from build123d import *

# Parameters (mm, degrees)
BOSS_EXTRUDE1_DEPTH = 7.6
SKETCH2_W           = 36.6
SKETCH2_H           = 8
BOSS_EXTRUDE2_DEPTH = 7.4
SKETCH3_R           = 2
CUT_EXTRUDE1_DEPTH  = 81.259594442
SKETCH4_R           = 2
CUT_EXTRUDE2_DEPTH  = 80.210873622


with BuildPart() as part:
    # Sketch1 → Boss-Extrude1 (new body)
    with BuildSketch(Plane.XY):
        with BuildLine():
            Line((57.05, 42), (41.05, 42))
            Line((41.05, 42), (37, 46.05))
            Line((37, 46.05), (34, 46.05))
            Line((34, 46.05), (32.25, 44.718087488))
            Line((32.25, 44.718087488), (32.25, 25.468087488))
            ThreePointArc((32.25, 25.468087488), (24.422154993, 14.809809015), (11.91, 19.09))
            Line((11.91, 19.09), (10, 21))
            Line((10, 21), (5, 21))
            Line((5, 21), (0, 16))
            Line((0, 16), (0, 0))
            Line((0, 0), (27.4, 0))
            Line((27.4, 0), (27.4, -8))
            Line((27.4, -8), (64, -8))
            Line((64, -8), (64, 35.05))
            Line((64, 35.05), (57.05, 42))
        make_face()
    extrude(amount=BOSS_EXTRUDE1_DEPTH)

    # Sketch2 → Boss-Extrude2 (add)
    with BuildSketch(Plane.XY.offset(7.6)):
        with Locations((45.7, -4)):
            Rectangle(SKETCH2_W, SKETCH2_H)
    extrude(amount=BOSS_EXTRUDE2_DEPTH)

    # Sketch3 → Cut-Extrude1 (cut, through all)
    with BuildSketch(Plane(origin=(0, 0, 0), x_dir=(1, 0, 0), z_dir=(0, 1, 0))):
        with Locations(Location((54, -11, 0), (0, 0, 270))):
            Circle(SKETCH3_R)
        with Locations(Location((34, -11, 0), (0, 0, 270))):
            Circle(SKETCH3_R)
    extrude(amount=-CUT_EXTRUDE1_DEPTH, mode=Mode.SUBTRACT)

    # Sketch4 → Cut-Extrude2 (cut, through all)
    with BuildSketch(Plane.XY.offset(7.6)):
        with Locations((5.08, 9.968087488)):
            Circle(SKETCH4_R)
        with Locations((36.08, 40.968087488)):
            Circle(SKETCH4_R)
    extrude(amount=-CUT_EXTRUDE2_DEPTH, mode=Mode.SUBTRACT)


solid = part.part
Read the model definition and answer for the solid it produces. Units are mm, in the model's axes. A direction names the side the tool comes from. Coordinates: 2 decimals unless noted, no trailing zeros. Loops run counter-clockwise (first coordinate to the right, second up) from the corner with the lowest first, then second, coordinate; pieces in that order, holes last. Notation, with made-up numbers: (-36, 23) -> (-7, 23) arc R21 cw to (-7, 30) -> close; hole circle Ø2 at (32, 58.25). An arc over 180 degrees is marked (long way). Answer in a Markdown table with one row per item.
Item 1: A cutting plane is placed at C-C on z = 6. Determine the outline of the cut face in (x, y), plus the area to 3 significant figures.
Returned:
| item | result |
|---|---|
| outline | (0, 0) -> (27.4, 0) -> (27.4, -8) -> (64, -8) -> (64, 35.05) -> (57.05, 42) -> (41.05, 42) -> (37, 46.05) -> (34, 46.05) -> (32.25, 44.72) -> (32.25, 25.47) arc R11.17 cw to (11.91, 19.09) -> (10, 21) -> (5, 21) -> (0, 16) -> close; hole circle Ø4 at (5.08, 9.97); hole circle Ø4 at (36.08, 40.97) |
| area | 2,170 mm^2 |
Item 2: Straight lines are drawn through the part: line 1 along X through (y, z) = (-3, 11); line 2 along Y through (x, z) = (55.5, 7); line 3 along Y through (x, z) = (5.08, 2.25). For each, find the intervals that lie inside material, in ascending order. Write a range as [from, to].
Returned:
| item | result |
|---|---|
| line 1 | x = [27.4, 32], [36, 52], [56, 64] |
| line 2 | y = [-8, 42] |
| line 3 | y = [0, 7.97], [11.97, 21] |
Item 3: A cutting plane is placed at B-B on x = 35. Determine the outline of the cut face in (y, z), plus the area to 3 significant figures.
Returned:
| item | result |
|---|---|
| outline | (-8, 0) -> (39.28, 0) -> (39.28, 7.6) -> (0, 7.6) -> (0, 9.27) -> (-8, 9.27) -> close; (-8, 12.73) -> (0, 12.73) -> (0, 15) -> (-8, 15) -> close; (42.65, 0) -> (46.05, 0) -> (46.05, 7.6) -> (42.65, 7.6) -> close |
| area | 417 mm^2 |
Item 4: A cutting plane is placed at A-A on z = 11. Determine the outline of the cut face in (x, y), plus the area to 3 significant figures.
Returned:
| item | result |
|---|---|
| outline | (27.4, -8) -> (32, -8) -> (32, 0) -> (27.4, 0) -> close; (36, -8) -> (52, -8) -> (52, 0) -> (36, 0) -> close; (56, -8) -> (64, -8) -> (64, 0) -> (56, 0) -> close |
| area | 229 mm^2 |
Item 5: Each of these flat-tipped pins is pushed along its axis until it touches: P1, Ø4.5, axis at x = 34, z = 11, coming from the -Y side; P2, Ø1.5, axis at x = 7.5, z = 4.5, coming from the +Y side; P3, Ø2, axis at x = 42, z = 10, coming from the +Y side; P4, Ø6, axis at x = 49.5, z = 5, coming from the +Y side. Where does it stop, or does it pass through?
Returned:
| item | result |
|---|---|
| P1 | stops at y = -8 |
| P2 | stops at y = 21 |
| P3 | stops at y = 0 |
| P4 | stops at y = 42 |
Item 6: For a pull along X with two mould halves and no side action, classify faces 6 (the cylindrical face through (4.82, 11.95, 3.85)), 7 (the flat face through (3, 19, 4)), 8 (the cylindrical face through (32, -4, 11)), 9 (the flat face through (60.57, 38.48, 3.75)) as released by +X, released by -X, zero draft, split by the parting line, or undercut.
Returned:
| item | result |
|---|---|
| face 6 | undercut |
| face 7 | released by -X |
| face 8 | undercut |
| face 9 | released by +X |
Item 7: A cutting plane is placed at D-D on y = 32. Determine the outline of the cut face in (x, z).
Returned:
| item | result |
|---|---|
| outline | (32.25, 0) -> (64, 0) -> (64, 7.6) -> (32.25, 7.6) -> close |
Item 8: For faces 1 (the flat face through (45, 0, 11)), 2 (the flat face through (27.4, -4, 7)), 3 (the flat face through (39, 13, 0)), 4 (the flat face through (11, 20, 4)), 5 (the flat face through (8, 21, 4)), determine the directions among +Z, -Z, +X, -X, +Y, -Y from which every point of the face is accessible in a straight line to the end or side of a thin tool.
Returned:
| item | result |
|---|---|
| face 1 | +Z, +X, -X, +Y |
| face 2 | +Z, -Z, -X, -Y |
| face 3 | -Z, +X, -X, +Y, -Y |
| face 4 | +Z, -Z, +Y |
| face 5 | +Z, -Z, -X, +Y |
